Verification items for the finished model (mm, model axes). A direction names the side the tool comes from. Round coordinates to 2 decimals unless told otherwise and drop trailing zeros. Write each loop counter-clockwise with the first axis right and the second up, starting at its lowest first coordinate (ties: lowest second). Pieces come first, ordered by that corner, then holes. Notation, with made-up numbers: M 33.25,69 L 64.25,69 A25 ccw 64.25,85 Z; hole C 15.5,59.5 d8. An arc over 180 degrees is marked long. One line per item, written item: value. Start each with the question number.
Item 1: Gauge pin test, flat ends, axial feed: pin 1 (4 mm diameter, centred on x = 15.5, y = -2.5, fed in from +Z); pin 2 (7.5 mm diameter, centred on x = 27, z = -18.5, fed in from -Y); pin 3 (4 mm diameter, centred on x = 35.5, y = -3.5, fed in from -Z); pin 4 (2 mm diameter, centred on x = -33.75, y = -3.5, fed in from +Z). Record the tip position at first contact, or that the pin passes through.
Item 2: Draft check along Z on faces 5 (the face through (-20.85, 2, 15)), 6 (the face through (0, -4, 0.85)), 7 (the face through (0, -2, 3.85)). Enter one of: +Z half, -Z half, draft (parallel to the pull), parting line (faces both ways), or undercut.
Item 3: Tool access check on faces 1 (the face through (-0.29, 6.01, 2.34)), 2 (the face through (35, -4, -2.85)), 3 (the face through (0, -2, -3.85)), 4 (the face through (25, 1, -18)). Record the directions out of +Z, -Z, +X, -X, +Y, -Y that give a thin tool (end or side, any length) a straight path to the whole face; none if there is none.
Item 4: Thickness scan on probe 1 along Z at (x, y) = (28, -4); probe 2 along X at (y, z) = (1.25, 23); probe 3 along Z at (x, y) = (0, -6). Record the ranges inside material, lowest first. Write a range as from..to.
Item 5: Section check C-C, the plane x = 13.5. Record the cut outline in (y, z).
Item 6: Section check D-D, the plane y = 2.75. Record the cut outline in (x, z).
Item 7: Section check B-B, the plane z = 10. Record the cut outline in (x, y).
Item 8: Section check A-A, the plane x = -33.75. Record the cut outline in (y, z).
from build123d import *

# Parameters (mm, degrees)
SKETCH1_W                = 60
SKETCH1_H                = 15
BOSS_EXTRUDE1_DEPTH      = 30
SKETCH2_W                = 60
SKETCH2_H                = 1.7
CUT_EXTRUDE1_DEPTH       = 8
SKETCH3_W                = 60
SKETCH3_H                = 1.8
CUT_EXTRUDE2_DEPTH       = 8.5
SKETCH4_W                = 60
SKETCH4_H                = 24
CUT_EXTRUDE3_DEPTH       = 3
SKETCH5_W                = 41.7
SKETCH5_H                = 24
CUT_EXTRUDE4_DEPTH       = 27
SKETCH6_W                = 60
SKETCH6_H                = 9.5
CUT_EXTRUDE5_DEPTH       = 8.5
SKETCH7_W                = 60
SKETCH7_H                = 17.5
CUT_EXTRUDE6_DEPTH       = 25
SKETCH9_W                = 9.15
SKETCH9_H                = 3
BOSS_EXTRUDE2_DEPTH      = 5
SKETCH10_W               = 41.7
SKETCH10_H               = 5.15
CUT_EXTRUDE7_DEPTH       = 23
CHAMFER1_SIZE            = 3
FILLET1_R                = 2
SKETCH11_W               = 7.5
SKETCH11_H               = 8
BOSS_EXTRUDE3_DEPTH      = 6
SKETCH12_R               = 1.9
CUT_EXTRUDE8_DEPTH       = 4
M2_CLEARANCE_HOLE1_D     = 2.2
M2_CLEARANCE_HOLE1_DEPTH = 10
SKETCH16_R               = 0.85
CUT_EXTRUDE9_DEPTH       = 81


with BuildPart() as part:
    # Sketch1 → Boss-Extrude1 (new body, symmetric)
    with BuildSketch(Plane.XY):
        Rectangle(SKETCH1_W, SKETCH1_H)
    extrude(amount=BOSS_EXTRUDE1_DEPTH, both=True)

    # Sketch2 → Cut-Extrude1 (cut)
    with BuildSketch(Plane.XZ.offset(7.5)):
        Rectangle(SKETCH2_W, SKETCH2_H)
    extrude(amount=-CUT_EXTRUDE1_DEPTH, mode=Mode.SUBTRACT)

    # Sketch3 → Cut-Extrude2 (cut)
    with BuildSketch(Plane.XZ.offset(7.5)):
        with Locations((0, -12.1)):
            Rectangle(SKETCH3_W, SKETCH3_H)
        with Locations((0, -23.4)):
            Rectangle(SKETCH3_W, SKETCH3_H)
    cut_extrude2 = extrude(amount=-CUT_EXTRUDE2_DEPTH, mode=Mode.SUBTRACT)

    # Sketch4 → Cut-Extrude3 (cut)
    with BuildSketch(Plane.XZ.offset(7.5)):
        with Locations((0, 18)):
            Rectangle(SKETCH4_W, SKETCH4_H)
    cut_extrude3 = extrude(amount=-CUT_EXTRUDE3_DEPTH, mode=Mode.SUBTRACT)

    # Sketch5 → Cut-Extrude4 (cut)
    with BuildSketch(Plane.XZ.offset(7.5)):
        with Locations((0, 18)):
            Rectangle(SKETCH5_W, SKETCH5_H)
    cut_extrude4 = extrude(amount=-CUT_EXTRUDE4_DEPTH, mode=Mode.SUBTRACT)

    # Sketch6 → Cut-Extrude5 (cut)
    with BuildSketch(Plane.XZ.offset(7.5)):
        with Locations((0, -17.75)):
            Rectangle(SKETCH6_W, SKETCH6_H)
    cut_extrude5 = extrude(amount=-CUT_EXTRUDE5_DEPTH, mode=Mode.SUBTRACT)

    # Sketch7 → Cut-Extrude6 (cut)
    with BuildSketch(Plane.XZ.offset(-1)):
        with Locations((0, -17.75)):
            Rectangle(SKETCH7_W, SKETCH7_H)
    cut_extrude6 = extrude(amount=CUT_EXTRUDE6_DEPTH, mode=Mode.SUBTRACT)

    # Mirror1: Cut-Extrude2, Cut-Extrude3, Cut-Extrude4, Cut-Extrude5, Cut-Extrude6 across plane
    add(cut_extrude2.mirror(Plane.XY), mode=Mode.SUBTRACT)
    add(cut_extrude3.mirror(Plane.XY), mode=Mode.SUBTRACT)
    add(cut_extrude4.mirror(Plane.XY), mode=Mode.SUBTRACT)
    add(cut_extrude5.mirror(Plane.XY), mode=Mode.SUBTRACT)
    add(cut_extrude6.mirror(Plane.XY), mode=Mode.SUBTRACT)

    # Sketch9 → Boss-Extrude2 (add)
    with BuildSketch(Plane.XZ.offset(7.5)):
        with Locations((-25.425, 7.5)):
            Rectangle(SKETCH9_W, SKETCH9_H)
        with Locations((-25.425, -7.5)):
            Rectangle(SKETCH9_W, SKETCH9_H)
        with Locations((25.425, -7.5)):
            Rectangle(SKETCH9_W, SKETCH9_H)
        with Locations((25.425, 7.5)):
            Rectangle(SKETCH9_W, SKETCH9_H)
    extrude(amount=-BOSS_EXTRUDE2_DEPTH)

    # Sketch10 → Cut-Extrude7 (cut)
    with BuildSketch(Plane.XZ.offset(7.5)):
        with Locations((0, 6.425)):
            Rectangle(SKETCH10_W, SKETCH10_H)
    cut_extrude7 = extrude(amount=-CUT_EXTRUDE7_DEPTH, mode=Mode.SUBTRACT)

    # Mirror2: Cut-Extrude7 across plane
    add(cut_extrude7.mirror(Plane.XY), mode=Mode.SUBTRACT)

    # Chamfer1
    chamfer1_edges = [part.edges().sort_by_distance(p)[0] for p in [
        (25.425, 7.5, 30),
        (-25.425, 7.5, -30),
        (0, 7.5, 3.85),
        (0, 7.5, -3.85),
        (25.425, 7.5, -30),
        (-25.425, 7.5, 30),
    ]]
    chamfer(chamfer1_edges, length=CHAMFER1_SIZE)

    # Fillet1
    fillet1_edges = [part.edges().sort_by_distance(p)[0] for p in [
        (0, 4.5, -3.85),
        (-25.425, 7.5, 27),
        (25.425, 7.5, 27),
        (25.425, 7.5, -27),
        (-25.425, 7.5, -27),
        (0, 7.5, 0.85),
        (0, 7.5, -0.85),
        (0, 4.5, 3.85),
        (-25.425, 4.5, -30),
        (25.425, 4.5, -30),
        (25.425, 4.5, 30),
        (-25.425, 4.5, 30),
    ]]
    fillet(fillet1_edges, radius=FILLET1_R)

    # Sketch11 → Boss-Extrude3 (add)
    with BuildSketch(Plane.XY.offset(-0.85)):
        with Locations((-33.75, -3.5)):
            Rectangle(SKETCH11_W, SKETCH11_H)
        with Locations((33.75, -3.5)):
            Rectangle(SKETCH11_W, SKETCH11_H)
    extrude(amount=-BOSS_EXTRUDE3_DEPTH)

    # Sketch12 → Cut-Extrude8 (cut)
    with BuildSketch(Plane(origin=(0, 0, -6.85), x_dir=(-1, 0, 0), z_dir=(0, 0, -1))):
        with Locations((33.75, -3.5)):
            Circle(SKETCH12_R)
    cut_extrude8 = extrude(amount=-CUT_EXTRUDE8_DEPTH, mode=Mode.SUBTRACT)

    # M2 Clearance Hole1
    with Locations(Plane(origin=(0, 0, -6.85), x_dir=(-1, 0, 0), z_dir=(0, 0, -1))):
        with Locations((33.75, -3.5)):
            m2_clearance_hole1 = Hole(M2_CLEARANCE_HOLE1_D / 2, depth=M2_CLEARANCE_HOLE1_DEPTH)

    # Mirror3: Cut-Extrude8, M2 Clearance Hole1 across plane
    add(cut_extrude8.mirror(Plane(origin=(0, 0, 0), x_dir=(0, 0, 1), z_dir=(1, 0, 0))), mode=Mode.SUBTRACT)
    add(m2_clearance_hole1.mirror(Plane(origin=(0, 0, 0), x_dir=(0, 0, 1), z_dir=(1, 0, 0))), mode=Mode.SUBTRACT)

    # Sketch16 → Cut-Extrude9 (cut)
    with BuildSketch(Plane.ZY.offset(37.5)):
        with Locations((0, 0.5)):
            Circle(SKETCH16_R)
    extrude(amount=-CUT_EXTRUDE9_DEPTH, mode=Mode.SUBTRACT)


solid = part.part
Response values:
1. pin 1: stops at z = 3.85
1. pin 2: stops at y = 1
1. pin 3: stops at z = -6.85
1. pin 4: passes through
2. face 5: draft
2. face 6: undercut
2. face 7: +Z half
3. face 1: +Z, +Y
3. face 2: -Z
3. face 3: -Z, +Y, -Y
3. face 4: +X, -X, -Y
4. probe 1: z = -30..-26.5, -9..-0.85, 0.85..9, 26.5..30
4. probe 2: x = -30..-20.85, 20.85..30
4. probe 3: z = -3.85..-0.85, 0.85..3.85
5. outline: M -7.5,-3.85 L 3.67,-3.85 A2 ccw 5.09,-3.26 L 6.91,-1.44 A2 ccw 7.5,-0.02 L 7.5,0.02 A2 ccw 6.91,1.44 L 5.09,3.26 A2 ccw 3.67,3.85 L -7.5,3.85 L -7.5,0.85 L 0.5,0.85 A0.85 cw 0.5,-0.85 L -7.5,-0.85 Z
6. outline: M -30,-30 L -20.85,-30 L -20.85,-3.85 L 20.85,-3.85 L 20.85,-30 L 30,-30 L 30,30 L 20.85,30 L 20.85,3.85 L -20.85,3.85 L -20.85,30 L -30,30 Z
7. outline: M -30,1 L -20.85,1 L -20.85,7.5 L -30,7.5 Z; M 20.85,1 L 30,1 L 30,7.5 L 20.85,7.5 Z
8. outline: M -7.5,-6.85 L -5.4,-6.85 L -5.4,-2.85 L -4.6,-2.85 L -4.6,-0.85 L -7.5,-0.85 Z; M -2.4,-2.85 L -1.6,-2.85 L -1.6,-6.85 L 0.5,-6.85 L 0.5,-0.85 L -2.4,-0.85 Z
